For this review, use the dimensioned drawing (mm, ordinates from the lowest corner) and the shaded views. A direction names the side the tool comes from. Round coordinates to 2 decimals unless told otherwise and drop trailing zeros. Order: outer loops, then holes, each group sorted by start corner. A loop starts at its lowest first (then second) coordinate and runs counter-clockwise, first axis right, second up. Notation, with made-up numbers: M 61,-7.75 L 119,-7.75 A10 cw 119,-3.75 Z; hole C 85,66.5 d11. An arc over 180 degrees is marked long. Answer as CSV lines item,"result". Start each with the question number.
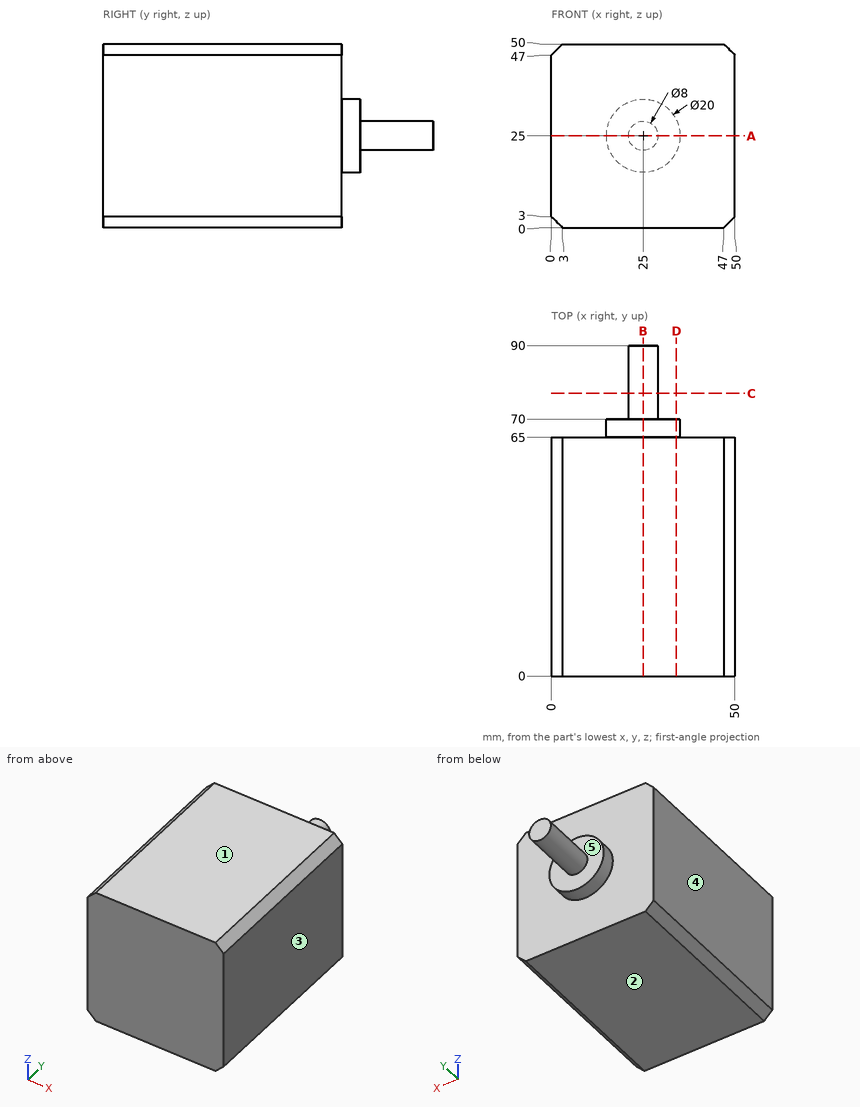
Item 1: Consider section B-B (x = 25). State the section outline as (y, z) points.
Item 2: For pin 1 (2 mm diameter, centred on y = 76.5, z = 21.5, fed in from +X); pin 2 (2 mm diameter, centred on x = 16.5, z = 23, fed in from +Y); pin 3 (8 mm diameter, centred on x = 20.5, y = 73, fed in from -Z), all flat-tipped, find the tip position at first contact; note any pin that passes through.
Item 3: Consider section A-A (z = 25). State the section outline as (x, y) points.
Item 4: Wall thickness on probe 1 along Y at (x, z) = (47.5, 6); probe 2 along Y at (x, z) = (31.5, 30.5); probe 3 along X at (y, z) = (78, 27.5): over which ranges is each line inside the solid? List them lowest first. Write a range as [from, to].
Item 5: Tool access review of the marked faces 4 and 5: name each direction out of +Z, -Z, +X, -X, +Y, -Y from which nothing blocks a thin tool from reaching the whole face with its end or side.
Item 6: The part is to be moulded in two halves that separate along Z. For the marked faces 1, 2 and 3, say which applies: +Z half, -Z half, draft (parallel to the pull), parting line (faces both ways), or undercut.
Item 7: Consider section C-C (y = 77). State the section outline as (x, z) points.
Item 8: Consider section D-D (x = 34). State the section outline as (y, z) points.
Reported:
1,outline,"M 0,0 L 65,0 L 65,15 L 70,15 L 70,21 L 90,21 L 90,29 L 70,29 L 70,35 L 65,35 L 65,50 L 0,50 Z"
2,pin 1,"stops at x = 28.12"
2,pin 2,"stops at y = 70"
2,pin 3,"stops at z = 15.17"
3,outline,"M 0,0 L 50,0 L 50,65 L 35,65 L 35,70 L 29,70 L 29,90 L 21,90 L 21,70 L 15,70 L 15,65 L 0,65 Z"
4,probe 1,"y = [0, 65]"
4,probe 2,"y = [0, 70]"
4,probe 3,"x = [21.88, 28.12]"
5,face 4,"+Z, -Z, -X, +Y, -Y"
5,face 5,"+Y"
6,face 1,"+Z half"
6,face 2,"-Z half"
6,face 3,"draft"
7,outline,"C 25,25 d8"
8,outline,"M 0,0 L 65,0 L 65,20.64 L 70,20.64 L 70,29.36 L 65,29.36 L 65,50 L 0,50 Z"
